from build123d import *

# Parameters (mm, degrees)
SKETCH_W     = 600
SKETCH_H     = 400
PAD_DEPTH    = 1200
POCKET_DEPTH = 400.001


with BuildPart() as part:
    # Sketch → Pad (new body)
    with BuildSketch(Plane.XZ):
        Rectangle(SKETCH_W, SKETCH_H)
    extrude(amount=PAD_DEPTH)

    # Sketch001 (on Face1 of Pad) → Pocket (cut, through all)
    with BuildSketch(Plane(origin=(0, 0, 200), x_dir=(-1, 0, 0), z_dir=(0, 0, 1))):
        with BuildLine():
            Line((-210, 900), (-210, 645))
            Line((-210, 645), (210, 645))
            Line((210, 900), (210, 645))
            ThreePointArc((210, 900), (0, 1110), (-210, 900))
        make_face()
        with BuildLine():
            ThreePointArc((-210, 300), (0, 90), (210, 300))
            Line((210, 555), (210, 300))
            Line((-210, 555), (210, 555))
            Line((-210, 555), (-210, 300))
        make_face()
    extrude(amount=-POCKET_DEPTH, mode=Mode.SUBTRACT)


solid = part.part
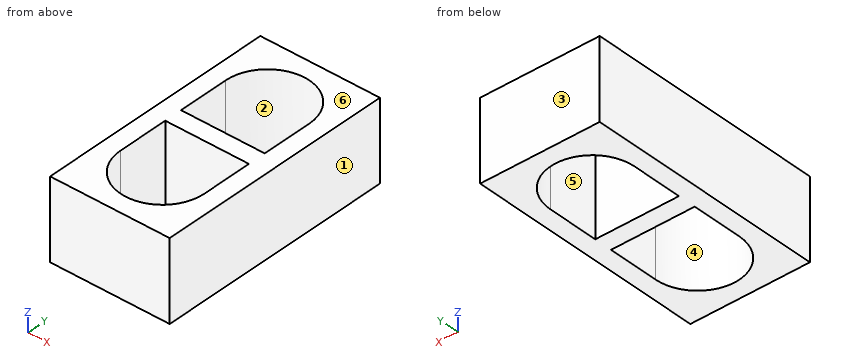
Part model, mm, in its own coordinate system. Face numbers are marked on the shaded views. A direction names the side the tool comes from. Give positions to 0.01 mm unless a question says otherwise; leave off trailing zeros. Order: outer loops, then holes, each group sorted by start corner. A loop starts at its lowest first (then second) coordinate and runs counter-clockwise, first axis right, second up. Notation, with made-up numbers: (17.25, 22.25) -> (28.25, 22.25) arc R25 ccw to (28.25, 39.25) -> close; hole circle Ø7 at (80.25, 48.5). An arc over 180 degrees is marked (long way). Use one line per item in the form item = value.
(1) Tool access for the marked faces 5 and 6: list every direction of +Z, -Z, +X, -X, +Y, -Y with a clear straight run to the whole face (end or side of a thin tool).
Solution:
face_5 = +Z, -Z
face_6 = +Z, +X, -X, +Y, -Y
(2) Saw through at D-D (y = -172). Write the cut outline in (x, z), then the cut area to 3 significant figures.
Solution:
outline = (-300, -200) -> (-166.48, -200) -> (-166.48, 200) -> (-300, 200) -> close; (166.48, -200) -> (300, -200) -> (300, 200) -> (166.48, 200) -> close
area = 107,000 mm²
(3) Saw through at A-A (x = 0). Write the cut outline in (y, z).
Solution:
outline = (-1200, -200) -> (-1110, -200) -> (-1110, 200) -> (-1200, 200) -> close; (-645, -200) -> (-555, -200) -> (-555, 200) -> (-645, 200) -> close; (-90, -200) -> (0, -200) -> (0, 200) -> (-90, 200) -> close
(4) Drill centre lines: line 1 (X direction, y = -714, z = -62); line 2 (Y direction, x = -164.5, z = -141); line 3 (Y direction, x = -94.5, z = 144.5). Where is each one in solid material? Low to high. Write a range as from..to.
Solution:
line_1 = -300..-210, 210..300
line_2 = -1200..-1030.54, -645..-555, -169.46..0
line_3 = -1200..-1087.54, -645..-555, -112.46..0
(5) Saw through at B-B (z = 170). Write the cut outline in (x, y), then the cut area to 3 significant figures.
Solution:
outline = (-300, -1200) -> (300, -1200) -> (300, 0) -> (-300, 0) -> close; hole (-210, -900) arc R210 ccw to (210, -900) -> (210, -645) -> (-210, -645) -> close; hole (-210, -555) -> (210, -555) -> (210, -300) arc R210 ccw to (-210, -300) -> close
area = 367,000 mm²
(6) Saw through at C-C (y = -880). Write the cut outline in (x, z).
Solution:
outline = (-300, -200) -> (-210, -200) -> (-210, 200) -> (-300, 200) -> close; (210, -200) -> (300, -200) -> (300, 200) -> (210, 200) -> close
(7) Flat gauge pin, fed straight in: P1, Ø2, axis at x = 164.5, z = -49.5, coming from the +Y side. Where does the tip first touch, or does it go through?
Solution:
P1 = 0
(8) Pull direction Y, two halves, no side cores. Call the marked faces 1, 2, 3 and 4: +Y half, -Y half, draft (parallel to the pull), parting line (faces both ways), or undercut.
Solution:
face_1 = draft
face_2 = undercut
face_3 = +Y half
face_4 = undercut
